```python
from build123d import *

# Parameters (mm, degrees)
SKETCH1_R           = 38.2
BOSS_EXTRUDE1_DEPTH = 180
SHELL1_T            = -2
CUT_EXTRUDE2_DEPTH  = 100


with BuildPart() as part:
    # Sketch1 → Boss-Extrude1 (new body)
    with BuildSketch(Plane(origin=(0, 0, 0), x_dir=(1, 0, 0), z_dir=(0, 1, 0))):
        with Locations(Location((0, 0, 0), (0, 0, 90))):
            Circle(SKETCH1_R)
    extrude(amount=BOSS_EXTRUDE1_DEPTH)

    # Shell1
    shell1_openings = [part.faces().sort_by_distance(p)[0] for p in [
        (0, 180, 0),
        (0, 0, 0),
    ]]
    offset(amount=SHELL1_T, openings=shell1_openings, kind=Kind.INTERSECTION)

    # Sketch4 → Cut-Extrude2 (cut)
    with BuildSketch(Plane(origin=(0, 10, 0), x_dir=(1, 0, 0), z_dir=(0, 1, 0))):
        with BuildLine():
            Line((0, 0), (14.618507116, 35.292198142))
            ThreePointArc((14.618507116, 35.292198142), (38.2, 0), (14.618507116, -35.292198142))
            Line((14.618507116, -35.292198142), (0, 0))
        make_face()
    extrude(amount=CUT_EXTRUDE2_DEPTH, mode=Mode.SUBTRACT)


solid = part.part
```
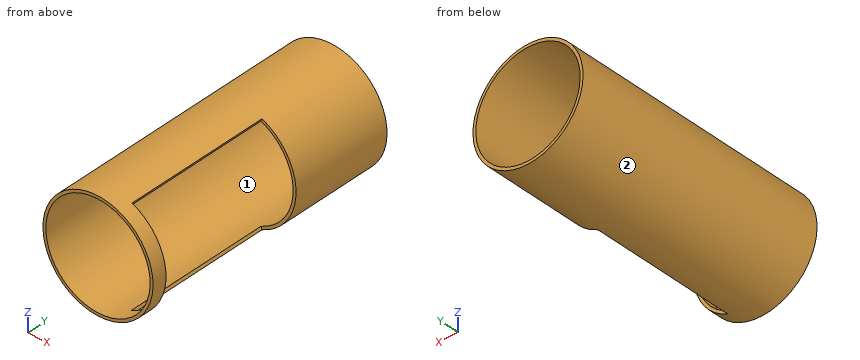
Build history of the part. All positions in model axes, mm. Face numbers are marked on the shaded views. Give positions to 0.01 mm unless a question says otherwise; leave off trailing zeros. Loops run counter-clockwise (first coordinate to the right, second up) from the corner with the lowest first, then second, coordinate; pieces in that order, holes last. Notation, with made-up numbers: (-2.5, 56) - (50.5, 56) arc R38 cw to (50.5, 95) - close; hole circle Ø10 at (34.25, 3.5). An arc over 180 degrees is marked (long way). Use a Markdown table: item, result.
(1) Band-saw the part on C-C (y = 124). Give the cut face in (x, z).
Taken from the geometry:
| item | result |
|---|---|
| outline | circle Ø76.4 at (0, 0); hole circle Ø72.4 at (0, 0) |
(2) Drop flat-ended pins along their axis: pin 1 Ø1.5 at (y, z) = (22.5, 27.5) entering from -X; pin 2 Ø12 at (y, z) = (82, 10) entering from -X; pin 3 Ø6 at (x, y) = (-23, 154) entering from -Z. Give the stop position or say it passes through.
Taken from the geometry:
| item | result |
|---|---|
| pin 1 | x = -27.27 |
| pin 2 | x = -37.99 |
| pin 3 | z = -32.55 |
(3) Band-saw the part on D-D (x = -34). Give the cut face in (y, z).
Taken from the geometry:
| item | result |
|---|---|
| outline | (0, -17.41) - (180, -17.41) - (180, -12.43) - (0, -12.43) - close; (0, 12.43) - (180, 12.43) - (180, 17.41) - (0, 17.41) - close |
(4) Band-saw the part on A-A (x = 0). Give the cut face in (y, z).
Taken from the geometry:
| item | result |
|---|---|
| outline | (0, -38.2) - (180, -38.2) - (180, -36.2) - (0, -36.2) - close; (0, 36.2) - (180, 36.2) - (180, 38.2) - (0, 38.2) - close |
(5) Band-saw the part on B-B (z = 0). Give the cut face in (x, y).
Taken from the geometry:
| item | result |
|---|---|
| outline | (-38.2, 0) - (-36.2, 0) - (-36.2, 180) - (-38.2, 180) - close; (36.2, 0) - (38.2, 0) - (38.2, 10) - (36.2, 10) - close; (36.2, 110) - (38.2, 110) - (38.2, 180) - (36.2, 180) - close |
(6) Pull direction X, two halves, no side cores. Call the marked faces 1 and 2: +X half, -X half, draft (parallel to the pull), parting line (faces both ways), or undercut.
Taken from the geometry:
| item | result |
|---|---|
| face 1 | undercut |
| face 2 | parting line |
(7) Wall check: line 1 along X through (y, z) = (134, 0); line 2 along Y through (x, z) = (29.5, 21.5); line 3 along X through (y, z) = (137, 4). Give the ranges that are in metal, low to high.
Taken from the geometry:
| item | result |
|---|---|
| line 1 | -38.2 to -36.2, 36.2 to 38.2 |
| line 2 | 0 to 10, 110 to 180 |
| line 3 | -37.99 to -35.98, 35.98 to 37.99 |
